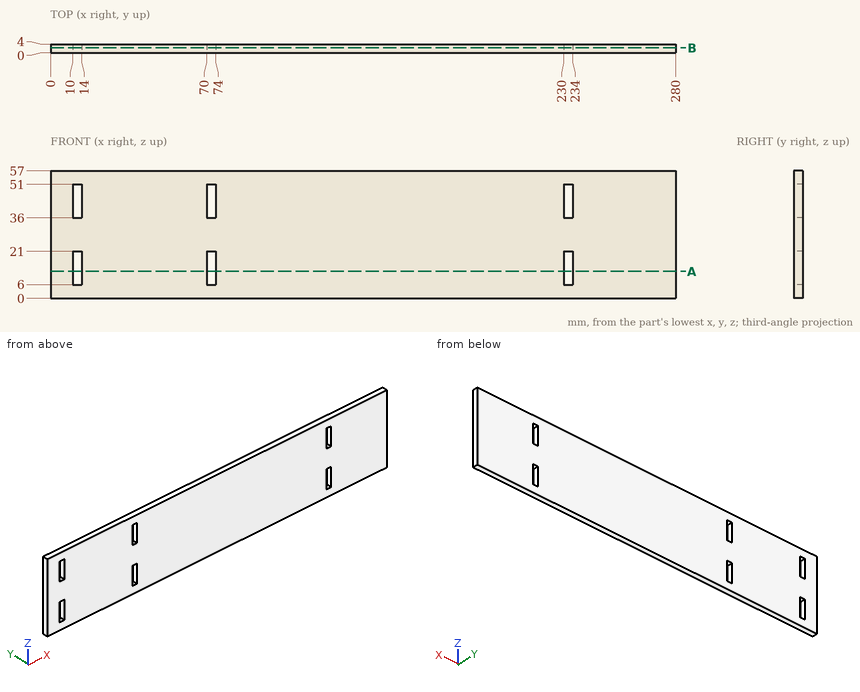
The figure shows three views and two pictorial views of one solid part (mm, origin at its lowest corner). Answer the questions. Coordinates: 2 decimals unless noted, no trailing zeros. Write each loop counter-clockwise with the first axis right and the second up, starting at its lowest first coordinate (ties: lowest second). Pieces come first, ordered by that corner, then holes. Notation, with made-up numbers: (-15.75, 27.5) -> (42.25, 27.5) arc R33 cw to (42.25, 56.5) -> close; hole circle Ø10 at (71, 53). An arc over 180 degrees is marked (long way). Return JSON: item names as keys, results as strings.
1. This flat-tipped pin is pushed along its axis until it touches: P1, Ø1, axis at y = 3, z = 32, coming from the -X side. Where does it stop, or does it pass through?
Found:
{"P1": "x = 0"}
2. Find the intervals of material crossed by line 1 along X through (y, z) = (1.55, 37); line 2 along Z through (x, y) = (231, 1.85), in increasing order. Write a range as from..to.
Found:
{"line 1": "0..10, 14..70, 74..230, 234..280", "line 2": "0..6, 21..36, 51..57"}
3. A cutting plane is placed at A-A (z = 12). Determine the outline of the cut face in (x, y).
Found:
{"outline": "(0, 0) -> (10, 0) -> (10, 4) -> (0, 4) -> close; (14, 0) -> (70, 0) -> (70, 4) -> (14, 4) -> close; (74, 0) -> (230, 0) -> (230, 4) -> (74, 4) -> close; (234, 0) -> (280, 0) -> (280, 4) -> (234, 4) -> close"}
4. A cutting plane is placed at B-B (y = 2.3). Determine the outline of the cut face in (x, z).
Found:
{"outline": "(0, 0) -> (280, 0) -> (280, 57) -> (0, 57) -> close; hole (10, 6) -> (14, 6) -> (14, 21) -> (10, 21) -> close; hole (10, 36) -> (14, 36) -> (14, 51) -> (10, 51) -> close; hole (70, 6) -> (74, 6) -> (74, 21) -> (70, 21) -> close; hole (70, 36) -> (74, 36) -> (74, 51) -> (70, 51) -> close; hole (230, 6) -> (234, 6) -> (234, 21) -> (230, 21) -> close; hole (230, 36) -> (234, 36) -> (234, 51) -> (230, 51) -> close"}
